```python
from build123d import *

# Parameters (mm, degrees)
SKETCH_W      = 169
SKETCH_H      = 98
PAD_DEPTH     = 5
SKETCH001_R   = 1.75
POCKET_DEPTH  = 5.001
FILLET_R      = 4
SKETCH002_R   = 7.5
SKETCH002_R_2 = 1.75
PAD001_DEPTH  = 5


with BuildPart() as part:
    # Sketch → Pad (new body)
    with BuildSketch(Plane.XY):
        Rectangle(SKETCH_W, SKETCH_H)
    extrude(amount=PAD_DEPTH)

    # Sketch001 (on Face6 of Pad) → Pocket (cut, through all)
    with BuildSketch(Plane.XY.offset(5)):
        with Locations((6, 39.5)):
            Circle(SKETCH001_R)
        with Locations((61, 39.5)):
            Circle(SKETCH001_R)
        with Locations((61, -39.5)):
            Circle(SKETCH001_R)
        with Locations((6, -39.5)):
            Circle(SKETCH001_R)
    extrude(amount=-POCKET_DEPTH, mode=Mode.SUBTRACT)

    # Fillet
    fillet_edges = [part.edges().sort_by_distance(p)[0] for p in [
        (-84.5, 49, 2.5),
        (-84.5, -49, 2.5),
        (84.5, -49, 2.5),
        (84.5, 49, 2.5),
    ]]
    fillet(fillet_edges, radius=FILLET_R)

    # Sketch002 (on Face5 of Pocket) → Pad001 (join)
    with BuildSketch(Plane.XY.offset(5)):
        with Locations((6, 39.5)):
            Circle(SKETCH002_R)
        with Locations((6, 39.5)):
            Circle(SKETCH002_R_2, mode=Mode.SUBTRACT)
        with Locations((61, 39.5)):
            Circle(SKETCH002_R)
        with Locations((61, 39.5)):
            Circle(SKETCH002_R_2, mode=Mode.SUBTRACT)
        with Locations((6, -39.5)):
            Circle(SKETCH002_R)
        with Locations((6, -39.5)):
            Circle(SKETCH002_R_2, mode=Mode.SUBTRACT)
        with Locations((61, -39.5)):
            Circle(SKETCH002_R)
        with Locations((61, -39.5)):
            Circle(SKETCH002_R_2, mode=Mode.SUBTRACT)
    extrude(amount=PAD001_DEPTH)


solid = part.part
```
Geometry check sheet. Reference: the model listing, model coordinates, mm. A direction names the side the tool comes from. Round coordinates to 2 decimals unless told otherwise and drop trailing zeros. Order: outer loops, then holes, each group sorted by start corner. A loop starts at its lowest first (then second) coordinate and runs counter-clockwise, first axis right, second up. Notation, with made-up numbers: (77, 58.5) -> (106, 58.5) arc R26 cw to (106, 79.5) -> close; hole circle Ø4 at (-5.5, -30). An arc over 180 degrees is marked (long way). Return JSON: item names as keys, results as strings. Group by question number.
Q1. Section check A-A, the plane y = -39.5. Record the boundary of the cut face in (x, z).
Q2. Material ranges on probe 1 along Y at (x, z) = (6, 7.7); probe 2 along Y at (x, z) = (60, 4.5); probe 3 along Z at (x, y) = (22.5, -22.5), recorded low to high. Write a range as from..to.
Q3. Release check for a two-part mould opening along X. For faces 3 (the cylindrical face through (-83.359, 47.797, 2.535)), 4 (the cylindrical face through (4.37, 32.18, 7.46)), 5 (the cylindrical face through (83.297, 47.859, 2.535)), 6 (the cylindrical face through (59.37, 32.18, 7.46)) record: released by +X, released by -X, zero draft, split by the parting line, or undercut.
Q4. Gauge pin test, flat ends, axial feed: pin 1 (2 mm diameter, centred on x = -36, y = 7, fed in from +Z); pin 2 (4 mm diameter, centred on x = 6, y = 39.5, fed in from -Z). Record the tip position at first contact, or that the pin passes through.
Q5. Tool access check on faces 1 (the flat face through (-1, 1, 5)), 2 (the flat face through (-1, 1, 0)). Record the directions out of +Z, -Z, +X, -X, +Y, -Y that give a thin tool (end or side, any length) a straight path to the whole face; none if there is none.
Q6. Section check B-B, the plane x = 61. Record the boundary of the cut face in (y, z), plus the area to 3 significant figures.
Q7. Section check D-D, the plane x = 43. Record the boundary of the cut face in (y, z), plus the area to 3 significant figures.
Q8. Section check C-C, the plane y = 23.5. Record the boundary of the cut face in (x, z).
Numbers:
{
 "1": {"outline": "(-84.5, 0) -> (4.25, 0) -> (4.25, 10) -> (-1.5, 10) -> (-1.5, 5) -> (-84.5, 5) -> close; (7.75, 0) -> (59.25, 0) -> (59.25, 10) -> (53.5, 10) -> (53.5, 5) -> (13.5, 5) -> (13.5, 10) -> (7.75, 10) -> close; (62.75, 0) -> (84.5, 0) -> (84.5, 5) -> (68.5, 5) -> (68.5, 10) -> (62.75, 10) -> close"},
 "2": {"probe 1": "-47..-41.25, -37.75..-32, 32..37.75, 41.25..47", "probe 2": "-49..-40.94, -38.06..38.06, 40.94..49", "probe 3": "0..5"},
 "3": {"face 3": "released by -X", "face 4": "undercut", "face 5": "released by +X", "face 6": "undercut"},
 "4": {"pin 1": "z = 5", "pin 2": "z = 0"},
 "5": {"face 1": "+Z", "face 2": "-Z, +X, -X, +Y, -Y"},
 "6": {"outline": "(-49, 0) -> (-41.25, 0) -> (-41.25, 10) -> (-47, 10) -> (-47, 5) -> (-49, 5) -> close; (-37.75, 0) -> (37.75, 0) -> (37.75, 10) -> (32, 10) -> (32, 5) -> (-32, 5) -> (-32, 10) -> (-37.75, 10) -> close; (41.25, 0) -> (49, 0) -> (49, 5) -> (47, 5) -> (47, 10) -> (41.25, 10) -> close", "area": "570 mm^2"},
 "7": {"outline": "(-49, 0) -> (49, 0) -> (49, 5) -> (-49, 5) -> close", "area": "490 mm^2"},
 "8": {"outline": "(-84.5, 0) -> (84.5, 0) -> (84.5, 5) -> (-84.5, 5) -> close"}
}
